Geometry: final body of the model. Coordinates: model frame, mm. A direction names the side the tool comes from. Coordinates: 2 decimals unless noted, no trailing zeros. Loops run counter-clockwise (first coordinate to the right, second up) from the corner with the lowest first, then second, coordinate; pieces in that order, holes last. Notation, with made-up numbers: (12, 22.5) - (34, 22.5) arc R29 ccw to (34, 50.5) - close; hole circle Ø3 at (8, 68). An arc over 180 degrees is marked (long way). Answer in a Markdown table with one row per item.
from build123d import *

# Parameters (mm, degrees)
F1_DEPTH = 495.3
F2_W     = 419.1
F2_H     = 406.4
F3_DEPTH = 532.497258


with BuildPart() as f1:
    # F0 (on Front) → F1 (new body)
    with BuildSketch(Plane.XZ):
        Polygon((-404.711319, 457.2), (-480.911319, 889), (-532.496258, 889), (-456.296258, 457.2), (-456.296258, 406.4), (-418.196258, 406.4), (-378.752236, 406.4), (-205.288432, 406.4), (-164.196258, 406.4), (-24.496258, 406.4), (-24.496258, 457.2), align=None)
        Polygon((0, 0), (-164.196258, 406.4), (-205.288432, 406.4), (-41.092174, 0), align=None)
        Polygon((-378.752236, 406.4), (-418.196258, 406.4), (-527.09081, 0), (-487.646788, 0), align=None)
    extrude(amount=F1_DEPTH)

    # F2 (on Right) → F3 (cut, through all)
    with BuildSketch(Plane.YZ):
        with Locations((-247.65, 203.2)):
            Rectangle(F2_W, F2_H)
    extrude(amount=-F3_DEPTH, mode=Mode.SUBTRACT)


solid = f1.part
(1) Cut plane A-A on z = 314. Output: boundary loops of the cut face in (x, y), then the cut area to 3 significant figures.
Verdict:
| item | result |
|---|---|
| outline | (-442.95, -495.3) - (-403.51, -495.3) - (-403.51, -457.2) - (-442.95, -457.2) - close; (-442.95, -38.1) - (-403.51, -38.1) - (-403.51, 0) - (-442.95, 0) - close; (-167.96, -495.3) - (-126.86, -495.3) - (-126.86, -457.2) - (-167.96, -457.2) - close; (-167.96, -38.1) - (-126.86, -38.1) - (-126.86, 0) - (-167.96, 0) - close |
| area | 6,140 mm² |
(2) First-contact query: pin 1 Ø12 at (x, y) = (-89, -408) entering from +Z; pin 2 Ø12 at (x, y) = (-240.5, -136.5) entering from -Z; pin 3 Ø15 at (y, z) = (-138, 423.5) entering from +X. Flat tips, straight axial feed; report the tip coordinate or a pass-through.
Verdict:
| item | result |
|---|---|
| pin 1 | stops at z = 457.2 |
| pin 2 | stops at z = 406.4 |
| pin 3 | stops at x = -24.5 |
(3) Cut plane D-D on z = 430. Output: boundary loops of the cut face in (x, y).
Verdict:
| item | result |
|---|---|
| outline | (-456.3, -495.3) - (-24.5, -495.3) - (-24.5, 0) - (-456.3, 0) - close |
(4) Pull-direction query (Y, two-part tool) for faces 1 (the face through (-433.96, -18.78, 200.36)), 2 (the face through (-327, 0, 414)), 3 (the face through (-102, -457.2, 202)); classes: pulls with the +Y half, pulls with the -Y half, needs draft (parallel to the pull), parting line crosses it, or undercut.
Verdict:
| item | result |
|---|---|
| face 1 | needs draft |
| face 2 | pulls with the +Y half |
| face 3 | undercut |
(5) Cut plane B-B on y = -82. Output: boundary loops of the cut face in (x, z).
Verdict:
| item | result |
|---|---|
| outline | (-532.5, 889) - (-456.3, 457.2) - (-456.3, 406.4) - (-24.5, 406.4) - (-24.5, 457.2) - (-404.71, 457.2) - (-480.91, 889) - close |
(6) Ray query, probe 1 along Y at (x, z) = (-492, 84.5); probe 2 along Z at (x, y) = (-182, -355.5); probe 3 along X at (y, z) = (-459, 258). Return the intervals inside material, ascending.
Verdict:
| item | result |
|---|---|
| probe 1 | y = -495.3 to -457.2, -38.1 to 0 |
| probe 2 | z = 406.4 to 457.2 |
| probe 3 | x = -457.96 to -418.52, -145.33 to -104.24 |
(7) Access query for faces 4 (the face through (-212, -244, 457.2)), 5 (the face through (-447, -38.1, 202)), 6 (the face through (-21, -476, 0)), 7 (the face through (-494.93, -244.18, 676.12)), 8 (the face through (-124.34, -475.983, 206.045)). Directions: +Z, -Z, +X, -X, +Y, -Y. A direction counts if a zero-diameter tool reaches every point of the face in a straight line with its end or side. Return the directions, or none.
Verdict:
| item | result |
|---|---|
| face 4 | +Z, +X, +Y, -Y |
| face 5 | -Z, +X, -X |
| face 6 | -Z, +X, -X, +Y, -Y |
| face 7 | -X, +Y, -Y |
| face 8 | -Z, +Y, -Y |
(8) Cut plane C-C on x = -354.5. Output: boundary loops of the cut face in (y, z).
Verdict:
| item | result |
|---|---|
| outline | (-495.3, 406.4) - (0, 406.4) - (0, 457.2) - (-495.3, 457.2) - close |
